Read the model definition and answer for the solid it produces. Units are mm, in the model's axes. Face numbers are marked on the shaded views. A direction names the side the tool comes from. Coordinates: 2 decimals unless noted, no trailing zeros. Write each loop counter-clockwise with the first axis right and the second up, starting at its lowest first coordinate (ties: lowest second). Pieces come first, ordered by that corner, then holes.
Item 1: Section A-A (z = 0) is taken. Give the vertices of the cut face in (x, y).
Item 2: A tool of negligible diameter and unlimited length cuts with its end or side. For the marked faces 4 and 5, from which of +Z, -Z, +X, -X, +Y, -Y can it reach the whole face along a straight path? Write none if from no direction.
Item 3: Determine the mould class of the marked faces 1, 2 and 3 for opening direction Z: released by +Z, released by -Z, zero draft, split by the parting line, or undercut.
Item 4: Section D-D (y = 6) is taken. Give the vertices of the cut face in (x, z).
Item 5: Each of these flat-tipped pins is pushed along its axis until it touches: P1, Ø5, axis at x = 0, z = 0, coming from the +Y side; P2, Ø3, axis at x = -5, y = 9, coming from the -Z side; P3, Ø2.5, axis at x = 0, z = 0, coming from the +Y side; P4, Ø1, axis at y = 8.5, z = -1.5, coming from the +X side. Where does it stop, or does it pass through?
Item 6: Straight lines are drawn through the part: probe 1 along Y at (x, z) = (1.25, 1); probe 2 along Y at (x, z) = (-6, 5.5); probe 3 along Z at (x, y) = (1.25, 3.5). For each, find the intervals that lie inside material, in ascending order.
Item 7: Section B-B (x = 0) is taken. Give the vertices of the cut face in (y, z).
Item 8: Section C-C (y = 9.5) is taken. Give the vertices of the cut face in (x, z), then the cut area to 3 significant figures.
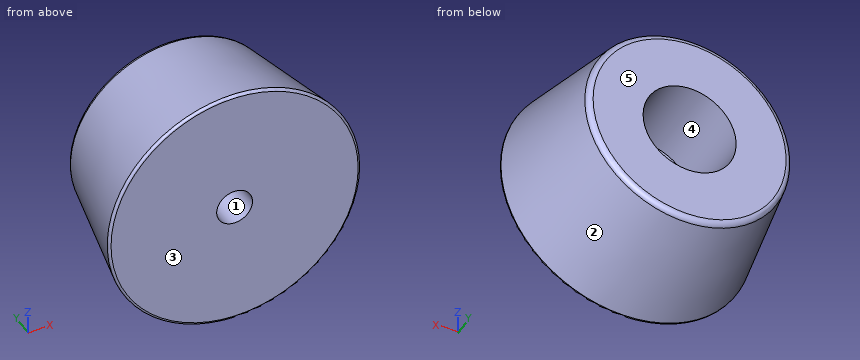
Autodesk Inventor part; units mm, degrees
ref_plane "YZ Plane" through (0, 0, 0) normal (1, 0, 0) x (0, 1, 0)
ref_plane "XZ Plane" through (0, 0, 0) normal (0, 1, 0) x (-1, 0, 0)
ref_plane "XY Plane" through (0, 0, 0) normal (0, 0, 1) x (1, 0, 0)
sketch "Эскиз1" plane through (0, 0, 0) normal (0, 0, 1) x (1, 0, 0)
  line L0 (0, 0) -> (0, 10.5)
  line L1 (3.9, 10.5) -> (8.5, 10.5)
  line L2 (8.5, 10.5) -> (10.6, 0)
  line L3 (0, 0) -> (10.6, 0)
  line L4 (3.9, 10.5) -> (3.9, 3.1378)
  line L5 (3.9, 3.1378) -> (1.5, 3.1378)
  line L6 (1.5, 3.1378) -> (1.5, 0)
  dimension "d0" = 10.5
  dimension "d1" = 3
  dimension "d2" = 7.8
  dimension "d3" = 17
  dimension "d4" = 21.2
revolve "Вращение1" add sketch "Эскиз1" angle 360 about axis through (0, 0, 0) along (0, 1, 0)
fillet "Сопряжение1" radius 0.2 1 edges at (-10.6, 0, 0)
fillet "Сопряжение2" radius 0.5 1 edges at (-8.5, 10.5, 0)
properties part number "ножки"
Established:
1. outline: (-10.55, 0.24) arc R0.2 ccw to (-10.36, 0) - (-1.5, 0) - (-1.5, 3.14) - (-3.9, 3.14) - (-3.9, 10.5) - (-8.09, 10.5) arc R0.5 ccw to (-8.58, 10.1) - close; (1.5, 0) - (10.36, 0) arc R0.2 ccw to (10.55, 0.24) - (8.58, 10.1) arc R0.5 ccw to (8.09, 10.5) - (3.9, 10.5) - (3.9, 3.14) - (1.5, 3.14) - close
2. face 4: +Y
2. face 5: +Z, -Z, +X, -X, +Y
3. face 1: undercut
3. face 2: split by the parting line
3. face 3: zero draft
4. outline: circle Ø18.8 at (0, 0); hole circle Ø7.8 at (0, 0)
5. P1: stops at y = 3.14
5. P2: stops at z = -8.15
5. P3: passes through
5. P4: stops at x = 8.9
6. probe 1: y = 0 to 3.14
6. probe 2: y = 0 to 10.5
6. probe 3: z = -9.82 to -3.69, 3.69 to 9.82
7. outline: (0, -10.36) arc R0.2 ccw to (0.24, -10.55) - (10.1, -8.58) arc R0.5 ccw to (10.5, -8.09) - (10.5, -3.9) - (3.14, -3.9) - (3.14, -1.5) - (0, -1.5) - close; (0, 1.5) - (3.14, 1.5) - (3.14, 3.9) - (10.5, 3.9) - (10.5, 8.09) arc R0.5 ccw to (10.1, 8.58) - (0.24, 10.55) arc R0.2 ccw to (0, 10.36) - close
8. outline: circle Ø17.4 at (0, 0); hole circle Ø7.8 at (0, 0)
8. area: 190 mm2
